```python
from build123d import *

# Parameters (mm, degrees)
SKETCH_1_W          = 9
SKETCH_1_H          = 6.5
EXTRUDE_1_DEPTH     = 112
SKETCH_2_R          = 1.75
CUT_EXTRUDE_2_DEPTH = 8
SKETCH_3_R          = 3
CUT_EXTRUDE_3_DEPTH = 3.5
CHAMFER_1_SIZE      = 0.5


with BuildPart() as part:
    # 草图1 → 拉伸1 (new body)
    with BuildSketch(Plane(origin=(0, 0, 0), x_dir=(0, 0, -1), z_dir=(1, 0, 0))):
        Rectangle(SKETCH_1_W, SKETCH_1_H)
    extrude(amount=EXTRUDE_1_DEPTH)

    # 草图2 → 拉伸2 (cut)
    with BuildSketch(Plane.XZ.offset(3.25)):
        with Locations(Location((7.5, 0, 0), (0, 0, 270))):
            Circle(SKETCH_2_R)
        with Locations((167.5, 0)):
            Circle(SKETCH_2_R)
        with Locations((187.5, 0)):
            Circle(SKETCH_2_R)
        with Locations((207.5, 0)):
            Circle(SKETCH_2_R)
        with Locations((227.5, 0)):
            Circle(SKETCH_2_R)
        with Locations((247.5, 0)):
            Circle(SKETCH_2_R)
        with Locations((267.5, 0)):
            Circle(SKETCH_2_R)
        with Locations((287.5, 0)):
            Circle(SKETCH_2_R)
        with Locations(Location((27.5, 0, 0), (0, 0, 270))):
            Circle(SKETCH_2_R)
        with Locations(Location((47.5, 0, 0), (0, 0, 270))):
            Circle(SKETCH_2_R)
        with Locations(Location((67.5, 0, 0), (0, 0, 270))):
            Circle(SKETCH_2_R)
        with Locations(Location((87.5, 0, 0), (0, 0, 270))):
            Circle(SKETCH_2_R)
        with Locations(Location((107.5, 0, 0), (0, 0, 270))):
            Circle(SKETCH_2_R)
        with Locations((127.5, 0)):
            Circle(SKETCH_2_R)
        with Locations((147.5, 0)):
            Circle(SKETCH_2_R)
    extrude(amount=-CUT_EXTRUDE_2_DEPTH, mode=Mode.SUBTRACT)

    # 草图3 → 拉伸3 (cut)
    with BuildSketch(Plane.XZ.offset(3.25)):
        with Locations(Location((7.5, 0, 0), (0, 0, 270))):
            Circle(SKETCH_3_R)
        with Locations((167.5, 0)):
            Circle(SKETCH_3_R)
        with Locations((187.5, 0)):
            Circle(SKETCH_3_R)
        with Locations((207.5, 0)):
            Circle(SKETCH_3_R)
        with Locations((227.5, 0)):
            Circle(SKETCH_3_R)
        with Locations((247.5, 0)):
            Circle(SKETCH_3_R)
        with Locations((267.5, 0)):
            Circle(SKETCH_3_R)
        with Locations((287.5, 0)):
            Circle(SKETCH_3_R)
        with Locations(Location((27.5, 0, 0), (0, 0, 270))):
            Circle(SKETCH_3_R)
        with Locations(Location((47.5, 0, 0), (0, 0, 270))):
            Circle(SKETCH_3_R)
        with Locations(Location((67.5, 0, 0), (0, 0, 270))):
            Circle(SKETCH_3_R)
        with Locations(Location((87.5, 0, 0), (0, 0, 270))):
            Circle(SKETCH_3_R)
        with Locations(Location((107.5, 0, 0), (0, 0, 270))):
            Circle(SKETCH_3_R)
        with Locations((127.5, 0)):
            Circle(SKETCH_3_R)
        with Locations((147.5, 0)):
            Circle(SKETCH_3_R)
    extrude(amount=-CUT_EXTRUDE_3_DEPTH, mode=Mode.SUBTRACT)

    # 倒角1
    chamfer_1_edges = [part.edges().sort_by_distance(p)[0] for p in [
        (56, 3.25, 4.5),
        (56, 3.25, -4.5),
        (56, -3.25, -4.5),
        (56, -3.25, 4.5),
    ]]
    chamfer(chamfer_1_edges, length=CHAMFER_1_SIZE)


solid = part.part
```
The model under review builds one solid part; all positions refer to its coordinate system, in mm. A direction names the side the tool comes from. Give positions to 0.01 mm unless a question says otherwise; leave off trailing zeros. Write each loop counter-clockwise with the first axis right and the second up, starting at its lowest first coordinate (ties: lowest second). Pieces come first, ordered by that corner, then holes. Notation, with made-up numbers: (-26, -36) -> (-10, -36) arc R12 ccw to (-10, -24) -> close; hole circle Ø1 at (88, -11.75). An arc over 180 degrees is marked (long way). Put each result on its own line as item: value.
(1) For pin 1 Ø3 at (x, z) = (47.5, 0) entering from -Y; pin 2 Ø3 at (x, z) = (8, 1) entering from -Y, all flat-tipped, find the tip position at first contact; note any pin that passes through.
Results are:
pin 1: through
pin 2: y = 0.25
(2) We need section B-B, the plane x = 67.5. Give the boundary of the cut face in (y, z).
Results are:
outline: (-3.25, -4) -> (-2.75, -4.5) -> (2.75, -4.5) -> (3.25, -4) -> (3.25, -1.75) -> (0.25, -1.75) -> (0.25, -3) -> (-3.25, -3) -> close; (-3.25, 3) -> (0.25, 3) -> (0.25, 1.75) -> (3.25, 1.75) -> (3.25, 4) -> (2.75, 4.5) -> (-2.75, 4.5) -> (-3.25, 4) -> close
(3) Tool access review of faces 4 (the cylindrical face through (29.235, 1.729, 0.228)), 5 (the cylindrical face through (84.57, -1.52, 0.65)): name each direction out of +Z, -Z, +X, -X, +Y, -Y from which nothing blocks a thin tool from reaching the whole face with its end or side.
Results are:
face 4: +Y, -Y
face 5: -Y
(4) To check wall thickness, follow probe 1 along Z at (x, y) = (87, 2.5); probe 2 along Z at (x, y) = (7, -1.25); probe 3 along Y at (x, z) = (66, -1.25). State the ranges of each line that lie inside material, in increasing order. Write a range as from..to.
Results are:
probe 1: -4.5..-1.68, 1.68..4.5
probe 2: -4.5..-2.96, 2.96..4.5
probe 3: 0.25..3.25
(5) The part is to be moulded in two halves that separate along Z. For faces 1 (the flat face through (55, 0, -4.5)), 2 (the flat face through (55, 0, 4.5)), 3 (the flat face through (45.5, 0.25, 0)), say which applies: pulls with the +Z half, pulls with the -Z half, needs draft (parallel to the pull), parting line crosses it, or undercut.
Results are:
face 1: pulls with the -Z half
face 2: pulls with the +Z half
face 3: undercut
(6) We need section A-A, the plane y = 1.5. Give the boundary of the cut face in (x, z).
Results are:
outline: (0, -4.5) -> (112, -4.5) -> (112, 4.5) -> (0, 4.5) -> close; hole circle Ø3.5 at (7.5, 0); hole circle Ø3.5 at (27.5, 0); hole circle Ø3.5 at (47.5, 0); hole circle Ø3.5 at (67.5, 0); hole circle Ø3.5 at (87.5, 0); hole circle Ø3.5 at (107.5, 0)
(7) We need section C-C, the plane z = 0. State how many separate pieces and enclosed holes the cut face has, and give its area (3 significant figures).
Results are:
separate pieces: 7
enclosed holes: 0
area: 539 mm²
